Read the model definition and answer for the solid it produces. Units are mm, in the model's axes. A direction names the side the tool comes from. Coordinates: 2 decimals unless noted, no trailing zeros. Loops run counter-clockwise (first coordinate to the right, second up) from the corner with the lowest first, then second, coordinate; pieces in that order, holes last.
Autodesk Inventor part; units mm, degrees
ref_plane "YZ Plane" through (0, 0, 0) normal (1, 0, 0) x (0, 1, 0)
ref_plane "XZ Plane" through (0, 0, 0) normal (0, 1, 0) x (-1, 0, 0)
ref_plane "XY Plane" through (0, 0, 0) normal (0, 0, 1) x (1, 0, 0)
sketch "Эскиз1" plane through (0, 0, 0) normal (0, 0, 1) x (1, 0, 0)
  arc A0 (-7.9205, 1.1252) -> (7.9205, 1.1252) centre (0, 0) ccw
  circle A1 centre (0, 14.2191) radius 6
  line L0 (7.9205, 1.1252) -> (5.9404, 15.0631)
  line L1 (-7.9205, 1.1252) -> (-5.9404, 15.0631)
  circle A2 centre (0, 0) radius 7
  arc A3 (7.9205, 1.1252) -> (-7.9205, 1.1252) centre (0, 0) ccw construction
  circle A4 centre (0, 14.2191) radius 2.5
  line L2 (2.3094, 18.2191) -> (4.6188, 14.2191)
  line L3 (4.6188, 14.2191) -> (2.3094, 10.2191)
  line L4 (2.3094, 10.2191) -> (-2.3094, 10.2191)
  line L5 (-2.3094, 10.2191) -> (-4.6188, 14.2191)
  line L6 (-4.6188, 14.2191) -> (-2.3094, 18.2191)
  line L7 (-2.3094, 18.2191) -> (2.3094, 18.2191)
  circle A5 centre (0, 0) radius 5
  point P0 (-5.6643, 4.1129)
  point P1 (-6.8918, 1.226)
  point P2 (-6.9958, -0.2431)
  point P3 (-5.2611, 17.1038)
  point P4 (-5.7507, 15.9307)
  point P5 (-5.9065, 15.2742)
extrude "Выдавливание1" add sketch "Эскиз1" against normal blind 2.5 contours L1 A1 L0 A0 | A1 | A2 | A4 | L2 L3 L4 L5 L6 L7 | A5
extrude "Выдавливание2" cut sketch "Эскиз1" against normal blind 1 contours A4
extrude "Выдавливание3" add sketch "Эскиз1" along normal blind 6 contours A1
extrude "Выдавливание4" add sketch "Эскиз1" along normal blind 0.5 contours L2 L3 L4 L5 L6 L7
extrude "Выдавливание5" add sketch "Эскиз1" along normal blind 10.5 contours A2
extrude "Выдавливание7" add sketch "Эскиз1" along normal blind 8.5 contours A5
properties part number "Капсула"
Item 1: A cutting plane is placed at B-B on x = 0. Determine the outline of the cut face in (y, z).
Numbers:
outline: (-8, -2.5) - (20.22, -2.5) - (20.22, 6) - (18.22, 6) - (18.22, 0.5) - (16.72, 0.5) - (16.72, -1) - (11.72, -1) - (11.72, 0.5) - (10.22, 0.5) - (10.22, 6) - (8.22, 6) - (8.22, 0) - (7, 0) - (7, 10.5) - (5, 10.5) - (5, 8.5) - (-5, 8.5) - (-5, 10.5) - (-7, 10.5) - (-7, 0) - (-8, 0) - close
Item 2: A cutting plane is placed at A-A on y = 0. Determine the outline of the cut face in (x, z), then the cut area to 3 significant figures.
Numbers:
outline: (-8, -2.5) - (8, -2.5) - (8, 0) - (7, 0) - (7, 10.5) - (5, 10.5) - (5, 8.5) - (-5, 8.5) - (-5, 10.5) - (-7, 10.5) - (-7, 0) - (-8, 0) - close
area: 167 mm2
Item 3: A cutting plane is placed at C-C on z = 9.5. Determine the outline of the cut face in (x, y).
Numbers:
outline: circle Ø14 at (0, 0); hole circle Ø10 at (0, 0)
Item 4: Determine the mould class of faces 3 (the face through (4, 16, 6)), 4 (the face through (0, 14, -1)), 5 (the face through (6.466, 2.681, 5.176)) for opening direction X: released by +X, released by -X, zero draft, split by the parting line, or undercut.
Numbers:
face 3: zero draft
face 4: undercut
face 5: split by the parting line
Item 5: A cutting plane is placed at D-D on y = 3.5. Determine the outline of the cut face in (x, z), then the cut area to 3 significant figures.
Numbers:
outline: (-7.58, -2.5) - (7.58, -2.5) - (7.58, 0) - (6.06, 0) - (6.06, 10.5) - (3.57, 10.5) - (3.57, 8.5) - (-3.57, 8.5) - (-3.57, 10.5) - (-6.06, 10.5) - (-6.06, 0) - (-7.58, 0) - close
area: 151 mm2
Item 6: Given pin 1 (4 mm diameter, centred on x = 4.5, z = 6, fed in from +Y); pin 2 (6 mm diameter, centred on y = -1, z = 8, fed in from -X); pin 3 (3 mm diameter, centred on x = 0, y = 14.22, fed in from +Z), each flat-ended and moving along its own axis, determine where each tip first touches the part or whether it passes through.
Numbers:
pin 1: stops at y = 19.67
pin 2: stops at x = -7
pin 3: stops at z = -1
Item 7: Find the intervals of material crossed by line 1 along Y through (x, z) = (-0.25, 4); line 2 along Y through (x, z) = (0, 10); line 3 along Y through (x, z) = (0, -0.2), in increasing order.
Numbers:
line 1: y = -7 to 7, 8.22 to 10.22, 18.22 to 20.21
line 2: y = -7 to -5, 5 to 7
line 3: y = -8 to 11.72, 16.72 to 20.22
Item 8: Which of the six approach directions +Z, -Z, +X, -X, +Y, -Y give full straight-line access (tool end or side, diameter ignored) to faces 1 (the face through (0, 6, -2.5)), 2 (the face through (3.48, 12.25, 3.21))?
Numbers:
face 1: -Z, +X, -X, +Y, -Y
face 2: +Z
